Part model, mm, in its own coordinate system. A direction names the side the tool comes from. Round coordinates to 2 decimals unless told otherwise and drop trailing zeros. Loops run counter-clockwise (first coordinate to the right, second up) from the corner with the lowest first, then second, coordinate; pieces in that order, holes last.
from build123d import *

# Parameters (mm, degrees)
BOX066_W                  = 10
BOX066_H                  = 4
BOX066_DEPTH              = 10
CYLINDER084_R             = 3
CYLINDER084_DEPTH         = 13
CYLINDER084_ROLL_ANGLE    = 90
CYLINDER087_R             = 1.25
CYLINDER087_DEPTH         = 22
CYLINDER087_PITCH_ANGLE   = 90
CYLINDER088_R             = 1.25
CYLINDER088_DEPTH         = 22
CYLINDER088_PITCH_ANGLE   = 90
CYLINDER086_R             = 1.25
CYLINDER086_DEPTH         = 22
CYLINDER086_PITCH_ANGLE   = 90
CYLINDER085_R             = 1.25
CYLINDER085_DEPTH         = 22
CYLINDER085_PITCH_ANGLE   = 90
FUSION063_ROLL_ANGLE      = 34
FUSION063_PLACEMENT_ANGLE = -90
FUSION064_ROLL_ANGLE      = 90
BOX065_W                  = 10
BOX065_H                  = 94
BOX065_DEPTH              = 4
BOX062_W                  = 14
BOX062_H                  = 3
BOX062_DEPTH              = 4
BOX061_W                  = 14
BOX061_H                  = 3
BOX061_DEPTH              = 4
BOX063_W                  = 14
BOX063_H                  = 3
BOX063_DEPTH              = 4
BOX064_W                  = 14
BOX064_H                  = 3
BOX064_DEPTH              = 4
SKETCH017_R               = 1.2
SKETCH017_W               = 24
SKETCH017_H               = 13
PAD012_DEPTH              = 140
CYLINDER080_R             = 6
CYLINDER080_DEPTH         = 31
CYLINDER080_ROLL_ANGLE    = 90
CYLINDER078_R             = 1.75
CYLINDER078_DEPTH         = 31
CYLINDER078_ROLL_ANGLE    = 90
BOX059_W                  = 17
BOX059_H                  = 77
BOX059_DEPTH              = 49
FILLET018013005_R         = 2
CYLINDER083_R             = 4
CYLINDER083_DEPTH         = 31
CYLINDER083_ROLL_ANGLE    = 90
CYLINDER079_R             = 1.75
CYLINDER079_DEPTH         = 31
CYLINDER079_ROLL_ANGLE    = 90
BOX058_W                  = 8
BOX058_H                  = 24
BOX058_DEPTH              = 11
BOX057_W                  = 76
BOX057_H                  = 76
BOX057_DEPTH              = 66
FILLET018013003_R         = 3.5
BOX060_W                  = 80
BOX060_H                  = 80
BOX060_DEPTH              = 63
FILLET018013006_R         = 1
CLONE024_PLACEMENT_ANGLE  = -90
SKETCH021_R               = 1
POCKET017_DEPTH           = 2


with BuildPart() as cubo012:
    # Box066 → Box066 (new body)
    with BuildSketch(Plane(origin=(-244, 64, 124), x_dir=(1, 0, 0), z_dir=(0, 0, 1))):
        with Locations((5, 2)):
            Rectangle(BOX066_W, BOX066_H)
    extrude(amount=BOX066_DEPTH)


with BuildPart() as cilindro019:
    # Cylinder084 → Cylinder084 (new body)
    with BuildSketch(Plane.XY):
        Circle(CYLINDER084_R)
    extrude(amount=CYLINDER084_DEPTH)


with BuildPart() as cilindro019_1:
    # Cylinder084 roll: moved
    add(cilindro019.part.rotate(Axis((0, 0, 0), (1, 0, 0)), CYLINDER084_ROLL_ANGLE))


with BuildPart() as cilindro019_2:
    # Cylinder084 placement: moved
    add(cilindro019_1.part.moved(Location((17.25, -6, 120))))


with BuildPart() as cilindro022:
    # Cylinder087 → Cylinder087 (new body)
    with BuildSketch(Plane.XY):
        Circle(CYLINDER087_R)
    extrude(amount=CYLINDER087_DEPTH)


with BuildPart() as cilindro022_1:
    # Cylinder087 pitch: moved
    add(cilindro022.part.rotate(Axis((0, 0, 0), (0, 1, 0)), CYLINDER087_PITCH_ANGLE))


with BuildPart() as cilindro022_2:
    # Cylinder087 placement: moved
    add(cilindro022_1.part.moved(Location((20.25, -38, 124.25))))


with BuildPart() as cilindro023:
    # Cylinder088 → Cylinder088 (new body)
    with BuildSketch(Plane.XY):
        Circle(CYLINDER088_R)
    extrude(amount=CYLINDER088_DEPTH)


with BuildPart() as cilindro023_1:
    # Cylinder088 pitch: moved
    add(cilindro023.part.rotate(Axis((0, 0, 0), (0, 1, 0)), CYLINDER088_PITCH_ANGLE))


with BuildPart() as cilindro023_2:
    # Cylinder088 placement: moved
    add(cilindro023_1.part.moved(Location((20.25, -26, 127.25))))


with BuildPart() as cilindro021:
    # Cylinder086 → Cylinder086 (new body)
    with BuildSketch(Plane.XY):
        Circle(CYLINDER086_R)
    extrude(amount=CYLINDER086_DEPTH)


with BuildPart() as cilindro021_1:
    # Cylinder086 pitch: moved
    add(cilindro021.part.rotate(Axis((0, 0, 0), (0, 1, 0)), CYLINDER086_PITCH_ANGLE))


with BuildPart() as cilindro021_2:
    # Cylinder086 placement: moved
    add(cilindro021_1.part.moved(Location((20.25, -30, 118.75))))


with BuildPart() as fusion064:
    # Cylinder085 → Cylinder085 (new body)
    with BuildSketch(Plane.XY):
        Circle(CYLINDER085_R)
    extrude(amount=CYLINDER085_DEPTH)


with BuildPart() as fusion064_1:
    # Cylinder085 pitch: moved
    add(fusion064.part.rotate(Axis((0, 0, 0), (0, 1, 0)), CYLINDER085_PITCH_ANGLE))


with BuildPart() as fusion064_2:
    # Cylinder085 placement: moved
    add(fusion064_1.part.moved(Location((20.25, -34, 132.75))))

    # Fusion063: union Cilindro022, Cilindro023, Cilindro021
    add(cilindro022_2.part)
    add(cilindro023_2.part)
    add(cilindro021_2.part)


with BuildPart() as fusion064_3:
    # Fusion063 roll: moved
    add(fusion064_2.part.rotate(Axis((0, 0, 0), (1, 0, 0)), FUSION063_ROLL_ANGLE))


with BuildPart() as fusion064_4:
    # Fusion063 placement: moved
    add(fusion064_3.part.moved(Location((114.107998, 21, 33.646227))).rotate(Axis((114.107998, 21, 33.646227), (0, 0, 1)), FUSION063_PLACEMENT_ANGLE))

    # Fusion064: union Cilindro019
    add(cilindro019_2.part)


with BuildPart() as fusion064_5:
    # Fusion064 roll: moved
    add(fusion064_4.part.rotate(Axis((0, 0, 0), (1, 0, 0)), FUSION064_ROLL_ANGLE))


with BuildPart() as fusion064_6:
    # Fusion064 placement: moved
    add(fusion064_5.part.moved(Location((-256.25, 172.75, 144))))


with BuildPart() as cubo:
    # Box065 → Box065 (new body)
    with BuildSketch(Plane(origin=(13, -11, 104), x_dir=(1, 0, 0), z_dir=(0, 0, 1))):
        with Locations((5, 47)):
            Rectangle(BOX065_W, BOX065_H)
    extrude(amount=BOX065_DEPTH)


with BuildPart() as cubo009:
    # Box062 → Box062 (new body)
    with BuildSketch(Plane(origin=(11, 75.5, 127), x_dir=(1, 0, 0), z_dir=(0, 0, 1))):
        with Locations((7, 1.5)):
            Rectangle(BOX062_W, BOX062_H)
    extrude(amount=BOX062_DEPTH)


with BuildPart() as cubo008:
    # Box061 → Box061 (new body)
    with BuildSketch(Plane(origin=(11, 75.5, 109), x_dir=(1, 0, 0), z_dir=(0, 0, 1))):
        with Locations((7, 1.5)):
            Rectangle(BOX061_W, BOX061_H)
    extrude(amount=BOX061_DEPTH)


with BuildPart() as cubo010:
    # Box063 → Box063 (new body)
    with BuildSketch(Plane(origin=(11, -6.5, 109), x_dir=(1, 0, 0), z_dir=(0, 0, 1))):
        with Locations((7, 1.5)):
            Rectangle(BOX063_W, BOX063_H)
    extrude(amount=BOX063_DEPTH)


with BuildPart() as cubo011:
    # Box064 → Box064 (new body)
    with BuildSketch(Plane(origin=(11, -6.5, 127), x_dir=(1, 0, 0), z_dir=(0, 0, 1))):
        with Locations((7, 1.5)):
            Rectangle(BOX064_W, BOX064_H)
    extrude(amount=BOX064_DEPTH)


with BuildPart() as pad012:
    # Sketch017 → Pad012 (new body)
    with BuildSketch(Plane(origin=(-0.25, -35, 0), x_dir=(1, 0, 0), z_dir=(0, -1, 0))):
        with Locations((37, 120)):
            Circle(SKETCH017_R)
        with Locations((9.5, 120)):
            Circle(SKETCH017_R)
        with Locations((23.25, 120)):
            Rectangle(SKETCH017_W, SKETCH017_H)
    extrude(amount=-PAD012_DEPTH)


with BuildPart() as cylinder107:
    # Cylinder080 → Cylinder080 (new body)
    with BuildSketch(Plane.XY):
        Circle(CYLINDER080_R)
    extrude(amount=CYLINDER080_DEPTH)


with BuildPart() as cylinder107_1:
    # Cylinder080 roll: moved
    add(cylinder107.part.rotate(Axis((0, 0, 0), (1, 0, 0)), CYLINDER080_ROLL_ANGLE))


with BuildPart() as cylinder107_2:
    # Cylinder080 placement: moved
    add(cylinder107_1.part.moved(Location((-4, 11, 83.5))))


with BuildPart() as cylinder105:
    # Cylinder078 → Cylinder078 (new body)
    with BuildSketch(Plane.XY):
        Circle(CYLINDER078_R)
    extrude(amount=CYLINDER078_DEPTH)


with BuildPart() as cylinder105_1:
    # Cylinder078 roll: moved
    add(cylinder105.part.rotate(Axis((0, 0, 0), (1, 0, 0)), CYLINDER078_ROLL_ANGLE))


with BuildPart() as cylinder105_2:
    # Cylinder078 placement: moved
    add(cylinder105_1.part.moved(Location((-8.5, 11, 71.5))))


with BuildPart() as fillet018013005:
    # Box059 → Box059 (new body)
    with BuildSketch(Plane(origin=(-14, -2.5, 75), x_dir=(1, 0, 0), z_dir=(0, 0, 1))):
        with Locations((8.5, 38.5)):
            Rectangle(BOX059_W, BOX059_H)
    extrude(amount=BOX059_DEPTH)

    # Fillet018013005
    fillet018013005_edges = [fillet018013005.edges().sort_by_distance(p)[0] for p in [
        (-14, -2.5, 99.5),
        (-14, 36, 124),
        (-14, 74.5, 99.5),
        (-14, 36, 75),
        (3, -2.5, 99.5),
        (3, 36, 124),
        (3, 74.5, 99.5),
        (3, 36, 75),
        (-5.5, -2.5, 75),
        (-5.5, -2.5, 124),
        (-5.5, 74.5, 75),
        (-5.5, 74.5, 124),
    ]]
    fillet(fillet018013005_edges, radius=FILLET018013005_R)


with BuildPart() as cylinder108:
    # Cylinder083 → Cylinder083 (new body)
    with BuildSketch(Plane.XY):
        Circle(CYLINDER083_R)
    extrude(amount=CYLINDER083_DEPTH)


with BuildPart() as cylinder108_1:
    # Cylinder083 roll: moved
    add(cylinder108.part.rotate(Axis((0, 0, 0), (1, 0, 0)), CYLINDER083_ROLL_ANGLE))


with BuildPart() as cylinder108_2:
    # Cylinder083 placement: moved
    add(cylinder108_1.part.moved(Location((-7, 80, 89.6))))


with BuildPart() as cylinder106:
    # Cylinder079 → Cylinder079 (new body)
    with BuildSketch(Plane.XY):
        Circle(CYLINDER079_R)
    extrude(amount=CYLINDER079_DEPTH)


with BuildPart() as cylinder106_1:
    # Cylinder079 roll: moved
    add(cylinder106.part.rotate(Axis((0, 0, 0), (1, 0, 0)), CYLINDER079_ROLL_ANGLE))


with BuildPart() as cylinder106_2:
    # Cylinder079 placement: moved
    add(cylinder106_1.part.moved(Location((-8.5, 80, 71.5))))


with BuildPart() as fusion061:
    # Box058 → Box058 (new body)
    with BuildSketch(Plane(origin=(-13.5, -13, 95), x_dir=(1, 0, 0), z_dir=(0, 0, 1))):
        with Locations((4, 12)):
            Rectangle(BOX058_W, BOX058_H)
    extrude(amount=BOX058_DEPTH)

    # Fusion061: union Cylinder107, Cylinder105, Fillet018013005, Cylinder108, Cylinder106
    add(cylinder107_2.part)
    add(cylinder105_2.part)
    add(fillet018013005.part)
    add(cylinder108_2.part)
    add(cylinder106_2.part)


with BuildPart() as fillet018013003:
    # Box057 → Box057 (new body)
    with BuildSketch(Plane(origin=(-21, -2, 87), x_dir=(1, 0, 0), z_dir=(0, 0, 1))):
        with Locations((38, 38)):
            Rectangle(BOX057_W, BOX057_H)
    extrude(amount=BOX057_DEPTH)

    # Fillet018013003
    fillet018013003_edges = [fillet018013003.edges().sort_by_distance(p)[0] for p in [
        (-21, -2, 120),
        (-21, 36, 153),
        (-21, 74, 120),
        (55, -2, 120),
        (55, 36, 153),
        (55, 74, 120),
        (17, -2, 153),
        (17, 74, 153),
    ]]
    fillet(fillet018013003_edges, radius=FILLET018013003_R)


with BuildPart() as fillet018013003_1:
    # Fillet018013003 placement: moved
    add(fillet018013003.part.moved(Location((0, 0, -24))))


with BuildPart() as body_more_holes:
    # Box060 → Box060 (new body)
    with BuildSketch(Plane(origin=(-23, -4, 68), x_dir=(1, 0, 0), z_dir=(0, 0, 1))):
        with Locations((40, 40)):
            Rectangle(BOX060_W, BOX060_H)
    extrude(amount=BOX060_DEPTH)

    # Cut103: cut Fillet018013003
    add(fillet018013003_1.part, mode=Mode.SUBTRACT)

    # Cut104: cut Fusion061
    add(fusion061.part, mode=Mode.SUBTRACT)

    # Cut105: cut Pad012
    add(pad012.part, mode=Mode.SUBTRACT)

    # Fusion062: union Cubo009, Cubo008, Cubo010, Cubo011
    add(cubo009.part)
    add(cubo008.part)
    add(cubo010.part)
    add(cubo011.part)

    # Fillet018013006
    fillet018013006_edges = [body_more_holes.edges().sort_by_distance(p)[0] for p in [
        (25, -6.5, 129),
        (11, -6.5, 129),
        (11, -6.5, 111),
        (25, -6.5, 111),
        (25, 78.5, 129),
        (11, 78.5, 129),
        (25, 78.5, 111),
        (11, 78.5, 111),
    ]]
    fillet(fillet018013006_edges, radius=FILLET018013006_R)

    # Cut107: cut Cubo
    add(cubo.part, mode=Mode.SUBTRACT)


with BuildPart() as body_more_holes_1:
    # Clone024 placement: moved
    add(body_more_holes.part.moved(Location((-275, 70, 2))).rotate(Axis((-275, 70, 2), (0, 0, 1)), CLONE024_PLACEMENT_ANGLE))

    # Cut108: cut Fusion064
    add(fusion064_6.part, mode=Mode.SUBTRACT)

    # Cut109: cut Cubo012
    add(cubo012.part, mode=Mode.SUBTRACT)

    # Sketch021 → Pocket017 (cut)
    with BuildSketch(Plane.XY.offset(133)):
        with Locations((-239, 59.25)):
            Circle(SKETCH021_R)
        with Locations((-232.5, 52.75)):
            Circle(SKETCH021_R)
        with Locations((-239, 46.25)):
            Circle(SKETCH021_R)
        with Locations((-245.5, 52.75)):
            Circle(SKETCH021_R)
    extrude(amount=-POCKET017_DEPTH, mode=Mode.SUBTRACT)


solid = body_more_holes_1.part
1) Slice it at C-C, the plane x = -268.5. Give the cut face in (y, z).
Values:
outline: (13, 70) - (15, 70) - (15, 127.5) arc R3.5 cw to (18.5, 131) - (87.5, 131) arc R3.5 cw to (91, 127.5) - (91, 70) - (93, 70) - (93, 133) - (13, 133) - close
2) Drop flat-ended pins along their axis: pin 1 Ø8 at (y, z) = (37, 77) entering from -X; pin 2 Ø10 at (y, z) = (73.5, 120.5) entering from +X; pin 3 Ø11 at (y, z) = (74, 85.5) entering from -X; pin 4 Ø2 at (y, z) = (60.75, 122) entering from -X. Give the stop position or say it passes through.
Values:
pin 1: stops at x = -279
pin 2: stops at x = -199
pin 3: stops at x = -200.56
pin 4: passes through
3) Slice it at B-B, the plane y = 33.25. Give the cut face in (x, z), then the cut area to 3 significant figures.
Values:
outline: (-279, 70) - (-277, 70) - (-277, 120.8) - (-279, 120.8) - close; (-279, 123.2) - (-277, 123.2) - (-277, 127.5) arc R3.5 cw to (-273.5, 131) - (-204.5, 131) arc R3.5 cw to (-201, 127.5) - (-201, 123.2) - (-199, 123.2) - (-199, 133) - (-279, 133) - close; (-201, 70) - (-199, 70) - (-199, 120.8) - (-201, 120.8) - close
area: 400 mm2
4) Tool access for faces 5 (the face through (-278, 47, 115.5)), 6 (the face through (-275.95, 90, 99.15)), 7 (the face through (-278, 80, 108)): list every direction of +Z, -Z, +X, -X, +Y, -Y with a clear straight run to the whole face (end or side of a thin tool).
Values:
face 5: +X, -X
face 6: -Z
face 7: -X
5) Wall check: line 1 along Y through (x, z) = (-239, 131.5); line 2 along Y through (x, z) = (-278, 122); line 3 along X through (y, z) = (17.5, 107). Give the ranges that are in metal, low to high.
Values:
line 1: y = 13 to 45.25, 47.25 to 49.75, 55.75 to 58.25, 60.25 to 64, 68 to 93
line 2: y = 13 to 32.05, 34.45 to 35, 59 to 59.55, 61.95 to 93
line 3: x = -279 to -276.85, -201.15 to -199
6) Mould opens along Z. For faces 1 (the face through (-278, 52, 110)), 2 (the face through (-199.74, 77.521, 95.566)), 3 (the face through (-246.237, 53.426, 132.014)), 4 (the face through (-198, 52, 111)) say: released by +Z, released by -Z, zero draft, split by the parting line, or undercut.
Values:
face 1: undercut
face 2: undercut
face 3: zero draft
face 4: released by -Z
7) Slice it at A-A, the plane z = 119.5. Give the cut face in (x, y).
Values:
outline: (-279, 13) - (-199, 13) - (-199, 35) - (-201, 35) - (-201, 18.5) arc R3.5 cw to (-204.5, 15) - (-273.5, 15) arc R3.5 cw to (-277, 18.5) - (-277, 35) - (-279, 35) - close; (-279, 59) - (-277, 59) - (-277, 67.68) arc R2 cw to (-277.5, 69) - (-277.5, 82) arc R2 cw to (-277, 83.32) - (-277, 87.5) arc R3.5 cw to (-273.5, 91) - (-204.5, 91) arc R3.5 cw to (-201, 87.5) - (-201, 83.32) arc R2 cw to (-200.5, 82) - (-200.5, 69) arc R2 cw to (-201, 67.68) - (-201, 59) - (-199, 59) - (-199, 93) - (-279, 93) - close
8) Slice it at D-D, the plane y = 21. Give the cut face in (x, z), then the cut area to 3 significant figures.
Values:
outline: (-279, 70) - (-277, 70) - (-277, 127.5) arc R3.5 cw to (-273.5, 131) - (-204.5, 131) arc R3.5 cw to (-201, 127.5) - (-201, 70) - (-199, 70) - (-199, 133) - (-279, 133) - close
area: 409 mm2
